```python
from build123d import *

# Parameters (mm, degrees)
PAD_DEPTH    = 20
PAD001_DEPTH = 17
PAD002_DEPTH = 7
SKETCH003_R  = 6
PAD003_DEPTH = 17


with BuildPart() as part:
    # Sketch → Pad (new body)
    with BuildSketch(Plane.XY):
        with BuildLine():
            Line((-137.2, 15), (137.2, 15))
            ThreePointArc((140, 12.2), (139.179899, 14.179899), (137.2, 15))
            Line((140, 12.2), (140, -12.2))
            ThreePointArc((137.2, -15), (139.179899, -14.179899), (140, -12.2))
            Line((137.2, -15), (-137.2, -15))
            ThreePointArc((-140, -12.2), (-139.179899, -14.179899), (-137.2, -15))
            Line((-140, -12.2), (-140, 12.2))
            ThreePointArc((-137.2, 15), (-139.179899, 14.179899), (-140, 12.2))
        make_face()
    extrude(amount=PAD_DEPTH)

    # Sketch001 → Pad001 (join)
    with BuildSketch(Plane.XY):
        with BuildLine():
            Line((20, 15), (22.1, 21.151423))
            ThreePointArc((22.1, 21.151423), (26.084071, 35.297898), (28.506759, 49.793628))
            ThreePointArc((28.506759, 49.793628), (28.121583, 67.94836), (23.000038, 85.369969))
            ThreePointArc((23.000038, 85.369969), (21.647561, 87.291244), (19.665958, 88.553679))
            ThreePointArc((19.665958, 88.553679), (12.226217, 90.931231), (4.547172, 92.357678))
            Line((4.547172, 92.357678), (-60.358943, 95.85))
            ThreePointArc((-60.358943, 95.85), (-62.26695, 95.75226), (-64.112729, 95.259163))
            ThreePointArc((-93.580829, 89.63501), (-78.596692, 91.136741), (-64.112729, 95.259163))
            ThreePointArc((-93.580829, 89.63501), (-94.676562, 89.247507), (-95.307077, 88.271167))
            Line((-95.307077, 88.271167), (-103.55, 58.933029))
            Line((-103.55, 58.933029), (-117.05, 58.933029))
            Line((-117.05, 58.933029), (-117.05, 141.429498))
            Line((-117.05, 141.429498), (-103.55, 141.429498))
            Line((-103.55, 141.429498), (-101.962901, 137.695318))
            ThreePointArc((-99.730837, 130.200634), (-100.635987, 134.010781), (-101.962901, 137.695318))
            ThreePointArc((-99.730837, 130.200634), (-98.973948, 128.771589), (-97.527521, 128.048472))
            ThreePointArc((-73.043885, 120.301604), (-84.988985, 125.112804), (-97.527521, 128.048472))
            ThreePointArc((-73.043885, 120.301604), (-62.760476, 119.837158), (-52.493885, 120.586391))
            ThreePointArc((-52.493885, 120.586391), (-15.446113, 126.09186), (21.410751, 132.756629))
            ThreePointArc((50.093063, 136.129962), (35.68651, 134.999351), (21.410751, 132.756629))
            ThreePointArc((83.803112, 94.973278), (77.196218, 123.945517), (50.093063, 136.129962))
            Line((83.803112, 94.973278), (68.949285, 33.703042))
            ThreePointArc((68.949285, 33.703042), (66.835565, 24.380889), (65, 15))
            Line((65, 15), (20, 15))
        make_face()
    extrude(amount=PAD001_DEPTH)

    # Sketch002 → Pad002 (join)
    with BuildSketch(Plane.XY):
        with BuildLine():
            Line((-114.376267, 58.938084), (-107.876267, 58.938084))
            Line((-107.876267, 31.188084), (-107.876267, 58.938084))
            Line((-106.176267, 31.188084), (-107.876267, 31.188084))
            Line((-106.176267, 31.188084), (-106.176267, 31.513084))
            ThreePointArc((-103.876267, 31.513084), (-105.026267, 32.663084), (-106.176267, 31.513084))
            Line((-103.876267, 31.513084), (-103.876267, 30.463084))
            ThreePointArc((-106.176267, 30.463084), (-105.026267, 29.313084), (-103.876267, 30.463084))
            Line((-106.176267, 30.463084), (-106.176267, 30.788084))
            Line((-107.876267, 30.788084), (-106.176267, 30.788084))
            Line((-107.876267, 26.938084), (-107.876267, 30.788084))
            Line((-110.826267, 26.938084), (-107.876267, 26.938084))
            Line((-110.826267, 19.138084), (-110.826267, 26.938084))
            Line((-111.126267, 17.821839), (-110.826267, 19.138084))
            Line((-111.426267, 19.138084), (-111.126267, 17.821839))
            Line((-111.426267, 26.938084), (-111.426267, 19.138084))
            Line((-114.376267, 26.938084), (-111.426267, 26.938084))
            Line((-114.376267, 32.538084), (-114.376267, 26.938084))
            Line((-115.926267, 32.538084), (-114.376267, 32.538084))
            Line((-115.926267, 32.538084), (-115.926267, 29.688084))
            ThreePointArc((-117.926267, 29.688084), (-116.926267, 28.688084), (-115.926267, 29.688084))
            Line((-117.926267, 36.188084), (-117.926267, 29.688084))
            ThreePointArc((-115.926267, 36.188084), (-116.926267, 37.188084), (-117.926267, 36.188084))
            Line((-115.926267, 36.188084), (-115.926267, 33.338084))
            Line((-115.926267, 33.338084), (-114.376267, 33.338084))
            Line((-114.376267, 58.938084), (-114.376267, 33.338084))
        make_face()
    extrude(amount=PAD002_DEPTH)

    # Sketch003 → Pad003 (join)
    with BuildSketch(Plane.XY):
        with BuildLine():
            ThreePointArc((118, 139.5), (105, 152.5), (92, 139.5))
            Line((92, 139.5), (92, 103.8))
            Line((83.55, 103.8), (92, 103.8))
            Line((83.55, 94.199976), (83.55, 103.8))
            Line((92, 94.199976), (83.55, 94.199976))
            Line((92, 58.499976), (92, 94.199976))
            ThreePointArc((92, 58.499976), (105.000012, 45.5), (118, 58.5))
            Line((118, 139.5), (118, 58.5))
        make_face()
        with Locations((105, 139.5)):
            Circle(SKETCH003_R, mode=Mode.SUBTRACT)
    extrude(amount=PAD003_DEPTH)


solid = part.part
```
Can you work these out from the model? Positions are in its coordinate system, mm. A direction names the side the tool comes from. Round coordinates to 2 decimals unless told otherwise and drop trailing zeros. Loops run counter-clockwise (first coordinate to the right, second up) from the corner with the lowest first, then second, coordinate; pieces in that order, holes last. Notation, with made-up numbers: (55.5, 30.25) -> (103.5, 30.25) arc R22 ccw to (103.5, 63.25) -> close; hole circle Ø2 at (-32, 77). An arc over 180 degrees is marked (long way). Answer in a Markdown table with one row per item.
Item 1: Will these pins go through, and if not, where does the flat tip stop? P1, Ø1.5, axis at y = 87, z = 8.5, coming from the -X side; P2, Ø1.4, axis at x = -107, z = 4, coming from the +Y side; P3, Ø3.5, axis at y = 23.5, z = 2.5, coming from the -X side.
Answer block:
| item | result |
|---|---|
| P1 | x = -117.05 |
| P2 | y = 141.43 |
| P3 | x = -111.43 |
Item 2: We'd pull the mould along X, two halves only. Please class faces 6 (the flat face through (2, -15, 10)), 7 (the cylindrical face through (12.332, 90.904, 8.381)), 8 (the flat face through (118, 100, 8)): released by +X, released by -X, zero draft, split by the parting line, or undercut.
Answer block:
| item | result |
|---|---|
| face 6 | zero draft |
| face 7 | undercut |
| face 8 | released by +X |
Item 3: On a 3-axis mill with a long thin cutter (end or side, diameter ignored), from which of +Z, -Z, +X, -X, +Y, -Y can I reach the whole of each face in a straight line? I mean faces 1 (the flat face through (25, 100, 17)), 2 (the flat face through (-112, 43, 7)), 3 (the cylindrical face through (-16, 126, 8)), 4 (the flat face through (-110.826, 23, 3)), 5 (the flat face through (-117.05, 100, 8)). Say none if no direction works.
Answer block:
| item | result |
|---|---|
| face 1 | +Z, +X, -X, +Y |
| face 2 | +Z, -X |
| face 3 | +Z, -Z, +Y |
| face 4 | +Z, -Z |
| face 5 | +Z, -Z, -X, +Y |
Item 4: If I drill on probe 1 along Y at (x, z) = (105, 8.75); probe 2 along X at (y, z) = (50, 5.5); probe 3 along Y at (x, z) = (-114, 2.75), over which ranges is the centre line in solid material (lowest first)?
Answer block:
| item | result |
|---|---|
| probe 1 | -15 to 15, 45.5 to 133.5, 145.5 to 152.5 |
| probe 2 | -114.38 to -107.88, 28.53 to 72.9, 95.16 to 114.84 |
| probe 3 | -15 to 15, 26.94 to 141.43 |
Item 5: Suppose I cut it at B-B, the plane y = 65.5. List the corners of the cut face in (x, z) for me.
Answer block:
| item | result |
|---|---|
| outline | (-117.05, 0) -> (-101.7, 0) -> (-101.7, 17) -> (-117.05, 17) -> close; (28.46, 0) -> (76.66, 0) -> (76.66, 17) -> (28.46, 17) -> close; (92, 0) -> (118, 0) -> (118, 17) -> (92, 17) -> close |
Item 6: Suppose I cut it at A-A, the plane x = 105. List the corners of the cut face in (y, z) for me.
Answer block:
| item | result |
|---|---|
| outline | (-15, 0) -> (15, 0) -> (15, 20) -> (-15, 20) -> close; (45.5, 0) -> (133.5, 0) -> (133.5, 17) -> (45.5, 17) -> close; (145.5, 0) -> (152.5, 0) -> (152.5, 17) -> (145.5, 17) -> close |
